```python
from build123d import *

# Parameters (mm, degrees)
EXTRUDE_1_DEPTH     = 39
SKETCH_3_R          = 9
CUT_EXTRUDE_1_DEPTH = 2
SKETCH_4_R          = 2.5
CUT_EXTRUDE_2_DEPTH = 10
CUT_EXTRUDE_4_DEPTH = 63.311796636


with BuildPart() as part:
    # 草图1 → 凸台-拉伸1 (new body)
    with BuildSketch(Plane(origin=(0, 0, 0), x_dir=(0, 0, -1), z_dir=(1, 0, 0))):
        with BuildLine():
            Line((0, 0), (10.409356218, 0))
            Line((10.409356218, 0), (15.75, 6.364731413))
            ThreePointArc((15.75, 6.364731413), (20, 16.6), (24.25, 6.364731413))
            Line((24.25, 6.364731413), (29.590643782, 0))
            Line((29.590643782, 0), (40, 0))
            Line((40, 0), (40, 27.6))
            Line((40, 27.6), (0, 27.6))
            Line((0, 27.6), (0, 0))
        make_face()
    extrude(amount=EXTRUDE_1_DEPTH)

    # 草图3 → 切除-拉伸1 (cut)
    with BuildSketch(Plane.ZY):
        with Locations((-20, 10.6)):
            Circle(SKETCH_3_R)
    cut_extrude_1 = extrude(amount=-CUT_EXTRUDE_1_DEPTH, mode=Mode.SUBTRACT)

    # 镜向1: 切除-拉伸1 across plane
    add(cut_extrude_1.mirror(Plane(origin=(19.5, 0, 0), x_dir=(0, 0, 1), z_dir=(1, 0, 0))), mode=Mode.SUBTRACT)

    # 草图4 → 切除-拉伸2 (cut)
    with BuildSketch(Plane(origin=(0, 27.6, 0), x_dir=(1, 0, 0), z_dir=(0, 1, 0))):
        with Locations(Location((6.5, 6, 0), (0, 0, 270))):
            Circle(SKETCH_4_R)
        with Locations(Location((6.5, 34, 0), (0, 0, 90))):
            Circle(SKETCH_4_R)
        with Locations(Location((32.5, 6, 0), (0, 0, 90))):
            Circle(SKETCH_4_R)
        with Locations(Location((32.5, 34, 0), (0, 0, 270))):
            Circle(SKETCH_4_R)
    extrude(amount=-CUT_EXTRUDE_2_DEPTH, mode=Mode.SUBTRACT)

    # 草图5 → 切除-拉伸4 (cut, through all)
    with BuildSketch(Plane.ZY):
        Polygon((0, 0), (-1.5, 0), (-1.5, 17.6), (0, 19.6), align=None)
        Polygon((-40, 19.6), (-40, 0), (-38.5, 0), (-38.5, 17.6), align=None)
    extrude(amount=-CUT_EXTRUDE_4_DEPTH, mode=Mode.SUBTRACT)


solid = part.part
```
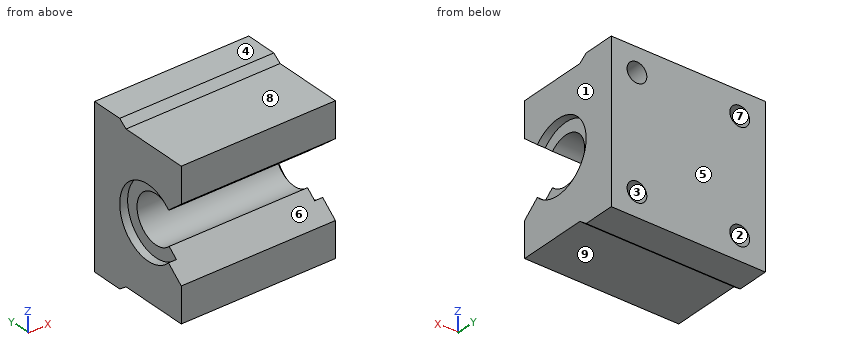
Could you check a few things on this model? Use its own coordinates, in mm. Face numbers are marked on the shaded views. A direction names the side the tool comes from. Round coordinates to 2 decimals unless told otherwise and drop trailing zeros. Loops run counter-clockwise (first coordinate to the right, second up) from the corner with the lowest first, then second, coordinate; pieces in that order, holes last.
Q1. I want a section at B-B (x = 5). Write out the boundary of the cut face in (y, z), and give its area (3 significant figures).
Q2. I want a section at C-C (z = -20). Write out the boundary of the cut face in (x, y).
Q3. On a 3-axis mill with a long thin cutter (end or side, diameter ignored), from which of +Z, -Z, +X, -X, +Y, -Y can I reach the whole of each face in a straight line? I mean the marked faces 5, 6, 7, 8 and 9. Say none if no direction works.
Q4. For P1, Ø1.5, axis at x = 5.5, z = -6.5, coming from the +Y side; P2, Ø1.5, axis at x = 16.5, y = 14.5, coming from the +Z side; P3, Ø12, axis at x = 9.5, y = 11.5, coming from the -Z side; P4, Ø11, axis at y = 10.6, z = -20, coming from the -X side, each with a flat end and sliding along its axis, tell me the tip position at first contact or that it passes through.
Q5. I want a section at D-D (y = 18.25). Write out the boundary of the cut face in (x, z).
Q6. Thinking about a two-plate mould opening in X: for the marked faces 1, 2, 3 and 4, which applies, pulls with the +X half, pulls with the -X half, needs draft (parallel to the pull), parting line crosses it, or undercut?
Q7. Please list where these lines run through material, in increasing order: L1, parallel to Z at x = 37.5, y = 10.6; L2, parallel to Z at x = 15.5, y = 10.6; L3, parallel to Z at x = 7.5, y = 25.75.
Q8. I want a section at A-A (y = 10.6). Write out the boundary of the cut face in (x, z).
Answer below:
1. outline: (0, -38.5) - (17.6, -38.5) - (19.6, -40) - (27.6, -40) - (27.6, -36) - (17.6, -36) - (17.6, -32) - (27.6, -32) - (27.6, -8) - (17.6, -8) - (17.6, -4) - (27.6, -4) - (27.6, 0) - (19.6, 0) - (17.6, -1.5) - (0, -1.5) - (0, -10.41) - (6.36, -15.75) arc R6 cw (long way) to (6.36, -24.25) - (0, -29.59) - close
1. area: 777 mm2
2. outline: (0, 19.6) - (2, 19.6) - (2, 16.6) - (37, 16.6) - (37, 19.6) - (39, 19.6) - (39, 27.6) - (0, 27.6) - close
3. face 5: +Z, -Z, +X, -X, +Y
3. face 6: +X, -X, -Y
3. face 7: +Y
3. face 8: +Z, +X, -X, -Y
3. face 9: -Z, +X, -X, -Y
4. P1: stops at y = 17.6
4. P2: stops at z = -1.5
4. P3: stops at z = -38.5
4. P4: passes through
5. outline: (0, -38.99) - (39, -38.99) - (39, -24.74) - (37, -24.74) - (37, -15.26) - (39, -15.26) - (39, -1.01) - (0, -1.01) - (0, -15.26) - (2, -15.26) - (2, -24.74) - (0, -24.74) - close; hole circle Ø5 at (6.5, -34); hole circle Ø5 at (6.5, -6); hole circle Ø5 at (32.5, -34); hole circle Ø5 at (32.5, -6)
6. face 1: pulls with the +X half
6. face 2: undercut
6. face 3: undercut
6. face 4: needs draft
7. L1: z = -38.5 to -29, -11 to -1.5
7. L2: z = -38.5 to -26, -14 to -1.5
7. L3: z = -40 to -36.29, -31.71 to -8.29, -3.71 to 0
8. outline: (0, -38.5) - (39, -38.5) - (39, -29) - (37, -29) - (37, -26) - (2, -26) - (2, -29) - (0, -29) - close; (0, -11) - (2, -11) - (2, -14) - (37, -14) - (37, -11) - (39, -11) - (39, -1.5) - (0, -1.5) - close
